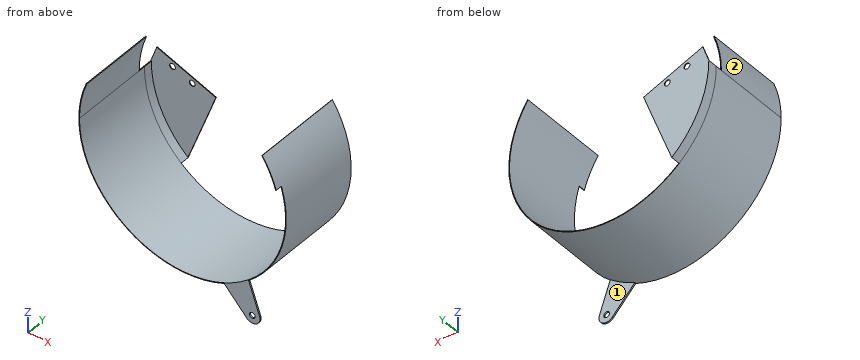
```python
from build123d import *
from build123d.topology import SkipClean

# Parameters (mm, degrees)
BASE_FLANGE1_DEPTH   = 102.87
CUT_EXTRUDE1_START   = -7.62
CUT_EXTRUDE1_DEPTH   = 7.62
BOSS_EXTRUDE5_START  = -95.25
BOSS_EXTRUDE5_DEPTH  = 95.25
BOSS_EXTRUDE6_DEPTH  = 10.16
BOSS_EXTRUDE7_DEPTH  = 0.762
SKETCH12_W           = 72.378245623
SKETCH12_H           = 0.762
BOSS_EXTRUDE8_DEPTH  = 20.33854962
SKETCH13_R           = 3.3
CUT_EXTRUDE2_DEPTH   = 204.597121983
SKETCH15_R           = 3.2639
BOSS_EXTRUDE10_DEPTH = 1.5875
BOSS_EXTRUDE11_START = 17.78
BOSS_EXTRUDE11_DEPTH = 87.63


# Read off the part's stored shape, not the designer's step: Cut-Extrude1
# Sheet-metal steps are written as plain solids
with BuildPart() as part:
    # Sketch2 → Base-Flange1 (new body)
    with BuildSketch(Plane(origin=(0, 0, 0), x_dir=(1, 0, 0), z_dir=(0, 1, 0))):
        with BuildLine():
            ThreePointArc((-119.38, 0), (35.898258345, 113.85472958), (97.790371047, -68.473554972))
            Line((97.790371047, -68.473554972), (97.186983651, -68.051058569))
            ThreePointArc((97.186983651, -68.051058569), (35.676758453, 113.152221674), (-118.6434, 0))
            Line((-118.6434, 0), (-119.38, 0))
        make_face()
    extrude(amount=BASE_FLANGE1_DEPTH)

    # Cut-Extrude1 outline → Cut-Extrude1 (cut)
    with BuildSketch(Plane.XZ.offset(CUT_EXTRUDE1_START)):
        with BuildLine():
            ThreePointArc((-119.38, 0), (18.160489843, -117.990597119), (113.85472958, 35.898258345))
            Line((113.85472958, 35.898258345), (113.152221674, 35.676758453))
            ThreePointArc((113.152221674, 35.676758453), (18.048435757, -117.262570031), (-118.6434, 0))
            Line((-118.6434, 0), (-119.38, 0))
        make_face()
    extrude(amount=CUT_EXTRUDE1_DEPTH, mode=Mode.SUBTRACT)

    # Sketch9 → Boss-Extrude5 (add)
    with BuildSketch(Plane(origin=(0, 102.87, 0), x_dir=(1, 0, 0), z_dir=(0, 1, 0)).offset(BOSS_EXTRUDE5_START)):
        with BuildLine():
            Line((-119.379693576, -0.270484204), (-118.6434, 0))
            Line((-118.6434, 0), (-119.38, 0))
            ThreePointArc((-119.38, 0), (-119.379923394, -0.135242189), (-119.379693576, -0.270484204))
        make_face()
    extrude(amount=BOSS_EXTRUDE5_DEPTH)

    # Sketch10 → Boss-Extrude6 (add)
    with SkipClean():  # the faces are left unmerged after this step: merging them gives an invalid solid
        with BuildSketch(Plane(origin=(0, 102.87, 0), x_dir=(1, 0, 0), z_dir=(0, 1, 0))):
            with BuildLine():
                Line((-119.379693576, -0.270484204), (-118.6434, 0))
                ThreePointArc((-118.6434, 0), (-107.527437301, 50.140867475), (-76.262507491, 90.886117283))
                Line((-76.262507491, 90.886117283), (-76.735984844, 91.45038562))
                ThreePointArc((-76.735984844, 91.45038562), (-108.252110006, 50.329564663), (-119.379693576, -0.270484204))
            make_face()
        extrude(amount=BOSS_EXTRUDE6_DEPTH)

    # Sketch11 → Boss-Extrude7 (add)
    with SkipClean():  # the faces are left unmerged after this step: merging them gives an invalid solid
        with BuildSketch(Plane(origin=(0, 113.03, 0), x_dir=(1, 0, 0), z_dir=(0, 1, 0))):
            with BuildLine():
                Line((-119.379693576, -0.270484204), (-51.440692331, 24.687531528))
                Line((-51.440692331, 24.687531528), (-76.735984844, 91.45038562))
                ThreePointArc((-76.735984844, 91.45038562), (-108.252110006, 50.329564663), (-119.379693576, -0.270484204))
            make_face()
        extrude(amount=BOSS_EXTRUDE7_DEPTH)

    # Sketch12 → Boss-Extrude8 (add)
    with SkipClean():  # the faces are left unmerged after this step: merging them gives an invalid solid
        with BuildSketch(Plane(origin=(-14.107419738, 0, -38.402251904), x_dir=(0.9386660406079884, 0, -0.3448275862069655), z_dir=(0.3448275862069655, 0, 0.9386660406079884))):
            with Locations((-75.961811901, 113.411)):
                Rectangle(SKETCH12_W, SKETCH12_H)
        extrude(amount=BOSS_EXTRUDE8_DEPTH)

    # Sketch13 → Cut-Extrude2 (cut, through all)
    with SkipClean():  # the faces are left unmerged after this step: merging them gives an invalid solid
        with BuildSketch(Plane(origin=(0, 113.792, 0), x_dir=(1, 0, 0), z_dir=(0, 1, 0))):
            with Locations(Location((-94.258662261, -5.860928581, 0), (0, 0, 270))):
                Circle(SKETCH13_R)
            with Locations(Location((-71.633967235, 2.450493285, 0), (0, 0, 270))):
                Circle(SKETCH13_R)
        extrude(amount=-CUT_EXTRUDE2_DEPTH, mode=Mode.SUBTRACT)

    # Sketch15 → Boss-Extrude10 (add)
    with SkipClean():  # the faces are left unmerged after this step: merging them gives an invalid solid
        with BuildSketch(Plane.XZ.offset(-7.62)):
            with BuildLine():
                Line((76.054879624, -92.017605302), (88.669451617, -127.404882133))
                ThreePointArc((88.669451617, -127.404882133), (84.957156503, -137.959730204), (73.860989671, -136.524099874))
                Line((73.860989671, -136.524099874), (47.938477772, -109.332002401))
                ThreePointArc((47.938477772, -109.332002401), (62.598204897, -101.651606695), (76.054879624, -92.017605302))
            make_face()
            with Locations(Location((80.295588053, -130.389929705, 0), (0, 0, 270))):
                Circle(SKETCH15_R, mode=Mode.SUBTRACT)
        extrude(amount=-BOSS_EXTRUDE10_DEPTH)

    # Sketch16 → Boss-Extrude11 (add)
    with SkipClean():  # the faces are left unmerged after this step: merging them gives an invalid solid
        with BuildSketch(Plane.XZ.offset(-113.03).offset(BOSS_EXTRUDE11_START)):
            with BuildLine():
                Line((-119.379693576, 0.270484204), (-118.6434, 0))
                ThreePointArc((-118.6434, 0), (-116.541899203, 22.231556259), (-110.311843526, 43.675548554))
                Line((-110.311843526, 43.675548554), (-110.896860103, 44.19808615))
                ThreePointArc((-110.896860103, 44.19808615), (-117.21446731, 22.635217102), (-119.379693576, 0.270484204))
            make_face()
        extrude(amount=BOSS_EXTRUDE11_DEPTH)


solid = part.part
```
Source: CAD feature listing. Evaluate the final solid. Frame: model axes, mm. Face numbers are marked on the shaded views. A direction names the side the tool comes from. Coordinates: 2 decimals unless noted, no trailing zeros. Loops run counter-clockwise (first coordinate to the right, second up) from the corner with the lowest first, then second, coordinate; pieces in that order, holes last. Notation, with made-up numbers: (87, 65) -> (96, 65) arc R22 ccw to (96, 89) -> close; hole circle Ø9 at (-9, -16). An arc over 180 degrees is marked (long way). One line per item, written item: value. Start each with the question number.
Q1. Section query A-A, the plane z = 14.5. Return the cut outline in (x, y), and give its area (3 significant figures).
Q2. Section query D-D, the plane x = 0. Return the cut outline in (y, z).
Q3. Section query C-C, the plane z = -61.5. Return the cut outline in (x, y), and give its area (3 significant figures).
Q4. Set-up query: the marked faces 1 and 2. Return all of +Z, -Z, +X, -X, +Y, -Y with unobstructed straight access to the full face (end or side cutting, diameter ignored); none if empty.
Q5. Contact query for flat-ended pins moving along their axis: P1, Ø1, axis at x = 30, y = 22.5, coming from the -Z side; P2, Ø1, axis at x = -43.5, y = 41, coming from the +Z side; P3, Ø2, axis at x = 60.5, y = 23.5, coming from the -Z side; P4, Ø4, axis at x = 87, z = -113.5, coming from the -Y side. Output: stop coordinate, or through.
Q6. Section query B-B, the plane y = 78.5. Return the cut outline in (x, z), and give its area (3 significant figures).
Q7. Line query: line 1 along X through (y, z) = (11, 1.5); line 2 along X through (y, z) = (96.5, -19); line 3 along Z through (x, y) = (102, 71.5). Output: solid intervals per line, ascending.
Results:
1. outline: (-118.5, 7.62) -> (-117.75, 7.62) -> (-117.75, 95.25) -> (-118.5, 95.25) -> close; (-114.15, 113.03) -> (-99.13, 113.03) -> (-99.13, 113.79) -> (-114.15, 113.79) -> close; (117.75, 7.62) -> (118.5, 7.62) -> (118.5, 102.87) -> (117.75, 102.87) -> close
1. area: 147 mm^2
2. outline: (7.62, -119.38) -> (102.87, -119.38) -> (102.87, -118.64) -> (7.62, -118.64) -> close
3. outline: (-102.32, 7.62) -> (-101.46, 7.62) -> (-101.46, 113.03) -> (-65.39, 113.03) -> (-65.39, 113.79) -> (-102.32, 113.79) -> close; (101.46, 7.62) -> (102.32, 7.62) -> (102.32, 102.87) -> (101.46, 102.87) -> close
3. area: 201 mm^2
4. face 1: -Z, +X, +Y
4. face 2: +Z, -X, +Y, -Y
5. P1: z = -115.68
5. P2: z = -110.18
5. P3: z = -103.5
5. P4: through
6. outline: (-119.38, 0) arc R119.38 ccw (long way) to (97.79, 68.47) -> (97.19, 68.05) arc R118.64 cw (long way) to (-110.31, 43.68) -> (-110.9, 44.2) arc R119.38 ccw to (-119.38, 0.27) arc R119.38 ccw to start
6. area: 362 mm^2
7. line 1: -119.37 to -118.63, 118.63 to 119.37
7. line 2: -117.86 to -117.11, 117.11 to 117.86
7. line 3: -62.03 to -60.6, 60.6 to 62.03
